Geometry: final body of the model. Coordinates: model frame, mm. Face numbers are marked on the shaded views. A direction names the side the tool comes from. Round coordinates to 2 decimals unless told otherwise and drop trailing zeros. Loops run counter-clockwise (first coordinate to the right, second up) from the corner with the lowest first, then second, coordinate; pieces in that order, holes last. Notation, with made-up numbers: (38, 5) - (70, 5) arc R25 ccw to (70, 33) - close; hole circle Ø5 at (-38, -31). An arc over 180 degrees is marked (long way). Answer as a JSON object with one key per item and string values. Group by question number.
Item 1: Draft query along Z for the marked faces 3, 4 and 5. Return one class per face: released by +Z, released by -Z, zero draft, split by the parting line, or undercut.
Item 2: First-contact query: pin 1 (1.5 mm diameter, centred on x = -20.5, y = -6.5, fed in from +Z); pin 2 (10 mm diameter, centred on x = 23.5, z = 46, fed in from +Y); pin 3 (5 mm diameter, centred on x = -31, z = 13.5, fed in from +Y); pin 4 (3 mm diameter, centred on x = -15.5, y = -6.5, fed in from +Z). Flat tips, straight axial feed; report the tip coordinate or a pass-through.
Item 3: Section C-C (x = -46.5). Return the cut outline in (y, z), plus the area to 3 significant figures.
Item 4: Reachability of the marked faces 1 and 2 from +Z, -Z, +X, -X, +Y, -Y: full face, straight path, thin tool, end or side. Return the list, or none.
Item 5: Section A-A (z = 28). Return the cut outline in (x, y), plus the area to 3 significant figures.
Item 6: Section B-B (y = -5). Count the separate pieces of the cut face and the enclosed holes in it, plus the area to 3 significant figures.
Item 7: Section D-D (x = 32.5). Return the cut outline in (y, z), plus the area to 3 significant figures.
Item 8: Line query: line 1 (Z direction, x = 0.5, y = -9); line 2 (X direction, y = -9.25, z = 60); line 3 (Z direction, x = -28.5, y = -8). Output: solid intervals per line, ascending.
```python
from build123d import *

# Parameters (mm, degrees)
F1_DEPTH = 10


with BuildPart() as f1:
    # F0 (on Front) → F1 (new body)
    with BuildSketch(Plane.XZ):
        with BuildLine():
            ThreePointArc((-55.31313, 17.172587), (-50.010384, 16.855003), (-45.055722, 14.938938))
            Line((-45.055722, 14.938938), (-42.555722, 19.269065))
            ThreePointArc((-42.555722, 19.269065), (-43.720537, 20.787081), (-43.470786, 22.684129))
            Line((-43.470786, 22.684129), (-21.970786, 59.923221))
            ThreePointArc((-21.970786, 59.923221), (-20.45277, 61.088036), (-18.555722, 60.838285))
            Line((-18.555722, 60.838285), (-16.055722, 65.168412))
            ThreePointArc((-16.055722, 65.168412), (-20.192413, 68.501242), (-23.118823, 72.934763))
            Line((-23.118823, 72.934763), (-24.715976, 70.168412))
            Line((-24.715976, 70.168412), (-53.715976, 19.938938))
            Line((-53.715976, 19.938938), (-55.31313, 17.172587))
        make_face()
        with BuildLine():
            ThreePointArc((-45.055722, 14.938938), (-38.741784, 8.625), (-36.430722, 0))
            Line((-36.430722, 0), (-31.430722, 0))
            ThreePointArc((-31.430722, 0), (-30.698489, 1.767767), (-28.930722, 2.5))
            Line((-28.930722, 2.5), (14.069278, 2.5))
            ThreePointArc((14.069278, 2.5), (15.837045, 1.767767), (16.569278, 0))
            Line((16.569278, 0), (21.569278, 0))
            ThreePointArc((21.569278, 0), (23.88034, 8.625), (30.194278, 14.938938))
            Line((30.194278, 14.938938), (27.694278, 19.269065))
            ThreePointArc((27.694278, 19.269065), (25.79723, 19.019314), (24.279214, 20.184129))
            Line((24.279214, 20.184129), (2.779214, 57.423221))
            ThreePointArc((2.779214, 57.423221), (2.529463, 59.320269), (3.694278, 60.838285))
            Line((3.694278, 60.838285), (1.194278, 65.168412))
            ThreePointArc((1.194278, 65.168412), (-7.430722, 62.85735), (-16.055722, 65.168412))
            Line((-16.055722, 65.168412), (-18.555722, 60.838285))
            ThreePointArc((-18.555722, 60.838285), (-17.640659, 59.923221), (-17.305722, 58.673221))
            ThreePointArc((-17.305722, 58.673221), (-17.390908, 58.026173), (-17.640659, 57.423221))
            Line((-17.640659, 57.423221), (-39.140659, 20.184129))
            ThreePointArc((-39.140659, 20.184129), (-40.658674, 19.019314), (-42.555722, 19.269065))
            Line((-42.555722, 19.269065), (-45.055722, 14.938938))
        make_face()
        with BuildLine():
            Line((-34.19515, 13.75), (-9.595786, 56.357349))
            ThreePointArc((-9.595786, 56.357349), (-7.430722, 57.607349), (-5.265659, 56.357349))
            Line((-5.265659, 56.357349), (19.333706, 13.75))
            ThreePointArc((19.333706, 13.75), (19.333706, 11.25), (17.168642, 10))
            Line((17.168642, 10), (-32.030087, 10))
            ThreePointArc((-32.030087, 10), (-34.19515, 11.25), (-34.19515, 13.75))
        make_face(mode=Mode.SUBTRACT)
        with BuildLine():
            Line((27.694278, 19.269065), (30.194278, 14.938938))
            ThreePointArc((30.194278, 14.938938), (35.14894, 16.855003), (40.451686, 17.172587))
            Line((40.451686, 17.172587), (8.257378, 72.934763))
            ThreePointArc((8.257378, 72.934763), (5.330969, 68.501242), (1.194278, 65.168412))
            Line((1.194278, 65.168412), (3.694278, 60.838285))
            ThreePointArc((3.694278, 60.838285), (5.591326, 61.088036), (7.109341, 59.923221))
            Line((7.109341, 59.923221), (12.294488, 50.942284))
            Line((12.294488, 50.942284), (28.609341, 22.684129))
            ThreePointArc((28.609341, 22.684129), (28.859092, 22.081176), (28.944278, 21.434129))
            ThreePointArc((28.944278, 21.434129), (28.609341, 20.184129), (27.694278, 19.269065))
        make_face()
        with BuildLine():
            ThreePointArc((-36.430722, 0), (-37.248692, -5.248895), (-39.625029, -10))
            Line((-39.625029, -10), (24.763585, -10))
            ThreePointArc((24.763585, -10), (22.387248, -5.248895), (21.569278, 0))
            Line((21.569278, 0), (16.569278, 0))
            ThreePointArc((16.569278, 0), (15.837045, -1.767767), (14.069278, -2.5))
            Line((14.069278, -2.5), (-28.930722, -2.5))
            ThreePointArc((-28.930722, -2.5), (-30.698489, -1.767767), (-31.430722, 0))
            Line((-31.430722, 0), (-36.430722, 0))
        make_face()
    extrude(amount=F1_DEPTH)


solid = f1.part
```
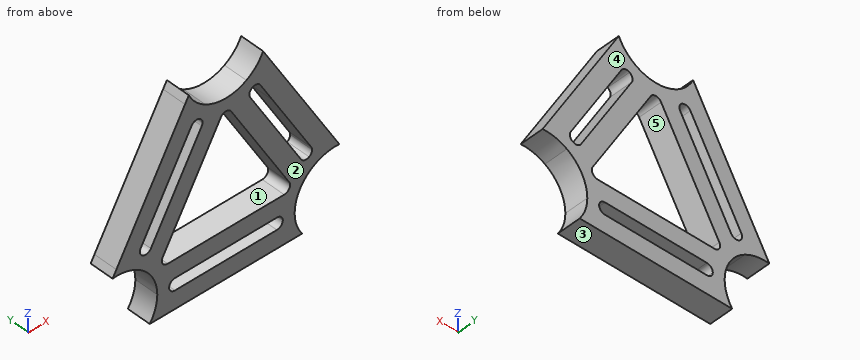
Values:
{
 "1": {"face 3": "released by -Z", "face 4": "zero draft", "face 5": "undercut"},
 "2": {"pin 1": "stops at z = 69.78", "pin 2": "stops at y = 0", "pin 3": "passes through", "pin 4": "stops at z = 65.75"},
 "3": {"outline": "(-10, 15.68) - (0, 15.68) - (0, 32.44) - (-10, 32.44) - close", "area": "168 mm^2"},
 "4": {"face 1": "+Y, -Y", "face 2": "+Z, -Z, +X, -X, -Y"},
 "5": {"outline": "(-49.06, -10) - (-40.4, -10) - (-40.4, 0) - (-49.06, 0) - close; (-34.63, -10) - (-25.97, -10) - (-25.97, 0) - (-34.63, 0) - close; (11.11, -10) - (19.77, -10) - (19.77, 0) - (11.11, 0) - close; (25.54, -10) - (34.2, -10) - (34.2, 0) - (25.54, 0) - close", "area": "346 mm^2"},
 "6": {"separate pieces": "1", "enclosed holes": "4", "area": "2,900 mm^2"},
 "7": {"outline": "(-10, 16.05) - (0, 16.05) - (0, 30.95) - (-10, 30.95) - close", "area": "149 mm^2"},
 "8": {"line 1": "z = -10 to -2.5, 2.5 to 10, 46.37 to 64.79", "line 2": "x = -30.59 to -21.92, -17.69 to 2.83, 7.06 to 15.73", "line 3": "z = -10 to -2.5, 2.5 to 10, 23.61 to 38.61, 48.61 to 63.61"}
}
